from build123d import *

# Parameters (mm, degrees)
SKETCH1_W               = 449.978341512
SKETCH1_H               = 427.573746213
BOSS_EXTRUDE1_DEPTH     = 378
DRAFT2_ANGLE            = 26
CUT_EXTRUDE1_DEPTH      = 854.283154982
CUT_EXTRUDE1_DEPTH_BACK = 854.283154982


with BuildPart() as part:
    # Sketch1 → Boss-Extrude1 (new body)
    with BuildSketch(Plane.XY):
        with Locations((224.989170756, 213.786873107)):
            Rectangle(SKETCH1_W, SKETCH1_H)
    extrude(amount=BOSS_EXTRUDE1_DEPTH)

    # Draft2
    draft2_faces = [part.faces().sort_by_distance(p)[0] for p in [
        (449.978341512, 213.786873106, 189),
    ]]
    draft(draft2_faces, Plane(origin=(0, 0, 0), x_dir=(-1, 0, 0), z_dir=(0, 0, -1)), DRAFT2_ANGLE)

    # Sketch2 → Cut-Extrude1 (cut, two sides: drawn at the far end of the back side and taken through both)
    with BuildSketch(Plane(origin=(0, 427.573746213, 0), x_dir=(1, 0, 0), z_dir=(0, 1, 0)).offset(-CUT_EXTRUDE1_DEPTH_BACK)):
        Polygon((-98.889763821, -1838.554406759), (12.856362316, -378), (18.603916927, -302.877787654), (526.667256984, -208.060368048), (556.854417648, -272.355099853), (580.648945558, -267.914441457), (2020.610369742, 0.818639262), (3940.798807951, -2211.804656514), (1821.298674388, -4051.177702535), align=None)
    extrude(amount=CUT_EXTRUDE1_DEPTH + CUT_EXTRUDE1_DEPTH_BACK, mode=Mode.SUBTRACT)


solid = part.part
Could you check a few things on this model? Use its own coordinates, in mm. A direction names the side the tool comes from. Give positions to 0.01 mm unless a question says otherwise; leave off trailing zeros. Loops run counter-clockwise (first coordinate to the right, second up) from the corner with the lowest first, then second, coordinate; pieces in that order, holes last. Notation, with made-up numbers: (25.5, 54.25) -> (69.5, 54.25) arc R23 ccw to (69.5, 69.25) -> close; hole circle Ø7 at (1.25, -20). An arc over 180 degrees is marked (long way). Return JSON: item names as keys, results as strings.
Item 1: I'm going to push flat-ended pins straight in: pin 1 (1.5 mm diameter, centred on y = 131, z = 259, fed in from +X); pin 2 (1 mm diameter, centred on x = 162, y = 318.5, fed in from +Z); pin 3 (1.5 mm diameter, centred on x = 313, y = 229, fed in from +Z). Where does each tip first touch, or does it pass through?
Geometry results:
{"pin 1": "stops at x = 576.67", "pin 2": "stops at z = 276.21", "pin 3": "stops at z = 248.08"}
Item 2: Which directions (+Z, -Z, +X, -X, +Y, -Y) give clear straight access to the entire face, cutting with the end or side of a thin tool? Please do faces 4 (the flat face through (269.079, 210.794, 256.133)), 5 (the flat face through (222, 217, 0)).
Geometry results:
{"face 4": "+Z, +Y, -Y", "face 5": "-Z, +X, -X, +Y, -Y"}
Item 3: If we section it at C-C on x = 494: List the corners of the cut face in (y, z) for me, plus the area to 3 significant figures.
Geometry results:
{"outline": "(0, 90.26) -> (427.57, 90.26) -> (427.57, 214.16) -> (0, 214.16) -> close", "area": "53,000 mm²"}
Item 4: If we section it at B-B on z = 249.5: List the corners of the cut face in (x, y) for me, plus the area to 3 significant figures.
Geometry results:
{"outline": "(0, 0) -> (304.62, 0) -> (304.62, 427.57) -> (0, 427.57) -> close; (546.12, 0) -> (571.67, 0) -> (571.67, 427.57) -> (546.12, 427.57) -> close", "area": "141,000 mm²"}
Item 5: If we section it at D-D on z = 346: List the corners of the cut face in (x, y) for me.
Geometry results:
{"outline": "(0, 0) -> (15.3, 0) -> (15.3, 427.57) -> (0, 427.57) -> close"}
Item 6: We'd pull the mould along X, two halves only. Please class faces 1 (the flat face through (568.585, 210.794, 270.166)), 2 (the flat face through (222, 427.574, 144)), 3 (the flat face through (541.55, 210.79, 239.76)): +X half, -X half, draft (parallel to the pull), parting line (faces both ways), or undercut.
Geometry results:
{"face 1": "+X half", "face 2": "draft", "face 3": "undercut"}
Item 7: I need wall thicknesses on L1, parallel to X at y = 190, z = 303.5; L2, parallel to Z at x = 91.5, y = 313.5; L3, parallel to X at y = 248, z = 362.5. Which ranges of each line are inside material? Lowest first, please. Write a range as from..to.
Geometry results:
{"L1": "x = 0..18.56", "L2": "z = 0..289.27", "L3": "x = 0..14.04"}
Item 8: If we section it at A-A on y = 161: List the corners of the cut face in (x, z) for me, plus the area to 3 significant figures.
Geometry results:
{"outline": "(0, 0) -> (449.98, 0) -> (580.65, 267.91) -> (556.85, 272.36) -> (526.67, 208.06) -> (18.6, 302.88) -> (12.86, 378) -> (0, 378) -> close", "area": "133,000 mm²"}
